For this review, take the finished solid that the model builds, in its own axes (mm). A direction names the side the tool comes from. Coordinates: 2 decimals unless noted, no trailing zeros. Return JSON: item names as keys, results as strings.
Autodesk Inventor part; units mm, degrees
ref_plane "YZ Plane" through (0, 0, 0) normal (1, 0, 0) x (0, 1, 0)
ref_plane "XZ Plane" through (0, 0, 0) normal (0, 1, 0) x (-1, 0, 0)
ref_plane "XY Plane" through (0, 0, 0) normal (0, 0, 1) x (1, 0, 0)
sketch "Sketch1" plane through (0, 0, 0) normal (0, 0, 1) x (1, 0, 0)
  line L0 (0, 0) -> (-6.35, 0)
  line L1 (0, 0) -> (0, 25.4)
  spline S0 degree 2 poles (-6.35, 0) (-6.2585, 13.0686) (0, 25.4) knots 0 0 0 1 1 1
  point P0 (-4.7625, 12.7)
  dimension "d0" = 6.35
  dimension "d1" = 25.4
revolve "Revolution1" add sketch "Sketch1" angle 360 about axis through (0, 0, 0) along (0, 1, 0)
sketch "Sketch2" plane through (0, 0, 0) normal (0, -1, 0) x (1, 0, 0)
  circle A0 centre (0, 0) radius 5.715
  dimension "d3" = 11.43
extrude "Extrusion1" add sketch "Sketch2" along normal blind 2.54
fillet "Fillet1" radius 2.54 1 edges at (-5.715, -2.54, 0)
properties part number "Rocket - Nose Cone"
1. Wall thickness on L1, parallel to X at y = -0.5, z = -4.5; L2, parallel to X at y = 7, z = -3; L3, parallel to Y at x = 2, z = 2.5: over which ranges is each line inside the solid? List them lowest first. Write a range as from..to.
Checks:
{"L1": "-3.44..3.44", "L2": "-5.02..5.02", "L3": "-2.54..17.93"}
2. Clearance check with flat-ended pins moving along their axes: pin 1 Ø5 at (x, y) = (-1.5, 15) entering from +Z; pin 2 Ø2 at (y, z) = (10, -3.5) entering from -X; pin 3 Ø4 at (x, z) = (1, 3.5) entering from +Y. State where each tip first meets the part, or that it passes through.
Checks:
{"pin 1": "z = 4.73", "pin 2": "x = -4.78", "pin 3": "y = 21.91"}
3. For faces 1 (the face through (6, 0, 1)), 2 (the face through (0, -2.54, 0)), list the 3-axis set-ups (+Z, -Z, +X, -X, +Y, -Y) from which the entire face can be reached by the end or side of a thin tool; tool diameter is ignored.
Checks:
{"face 1": "-Y", "face 2": "+Z, -Z, +X, -X, -Y"}
